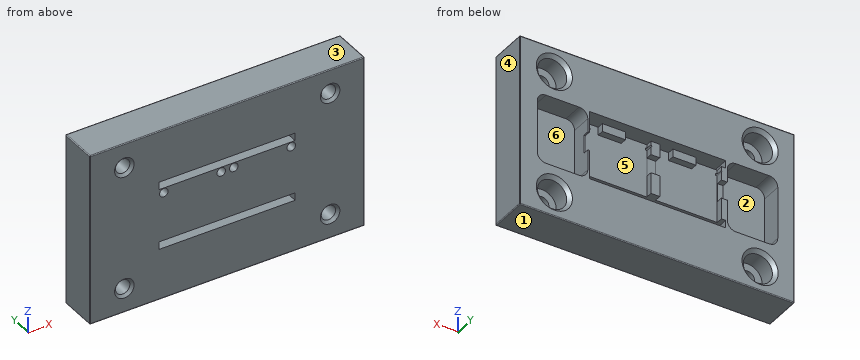
from build123d import *

# Parameters (mm, degrees)
SKETCH1_W             = 80.1116
SKETCH1_H             = 50.2158
BOSS_EXTRUDE1_DEPTH   = 11.176
HOLE1_D               = 4.191
HOLE1_CBORE_D         = 8.509
HOLE1_CBORE_DEPTH     = 5.7912
CHAMFER1_SIZE         = 1.016
FILLET1_R             = 0.254
CHAMFER2_SIZE         = 0.762
SKETCH4_W             = 39.751
SKETCH4_H             = 2.2352
CUT_EXTRUDE1_DEPTH    = 96.207132087
SKETCH5_R             = 1.2446
CUT_EXTRUDE2_DEPTH    = 4.2164
LPATTERN1_COUNT       = 2
LPATTERN1_PITCH       = 20.4216
F_1_0MM_DOWEL_HOLE1_D = 0.6858
SKETCH12_W            = 14.732
SKETCH12_H            = 20.32
CUT_EXTRUDE3_DEPTH    = 6.0198
FILLET2_R             = 2.54
CUT_EXTRUDE4_DEPTH    = 1.905
CUT_EXTRUDE5_REACH    = 81.263
SKETCH14_W            = 5.3848
SKETCH14_H            = 1.838231329


with BuildPart() as part:
    # Sketch1 → Boss-Extrude1 (new body)
    with BuildSketch(Plane(origin=(0, 0, 0), x_dir=(1, 0, 0), z_dir=(0, 1, 0))):
        with Locations((40.0558, 25.1079)):
            Rectangle(SKETCH1_W, SKETCH1_H)
    extrude(amount=BOSS_EXTRUDE1_DEPTH)

    # Hole1 (through all)
    with Locations(Plane(origin=(0, 11.176, 0), x_dir=(1, 0, 0), z_dir=(0, 1, 0))):
        with Locations((10.0457, 7.0993), (10.0584, 43.1419), (70.0532, 43.1292), (70.0532, 7.112)):
            CounterBoreHole(HOLE1_D / 2, HOLE1_CBORE_D / 2, HOLE1_CBORE_DEPTH)

    # Chamfer1
    chamfer1_edges = [part.edges().sort_by_distance(p)[0] for p in [
        (65.7987, 11.176, -7.112),
        (65.7987, 11.176, -43.1292),
        (5.8039, 11.176, -43.1419),
        (5.7912, 11.176, -7.0993),
    ]]
    chamfer(chamfer1_edges, length=CHAMFER1_SIZE)

    # Fillet1
    fillet1_edges = [part.edges().sort_by_distance(p)[0] for p in [
        (80.1116, 11.176, -25.1079),
        (40.0558, 11.176, -50.2158),
        (0, 11.176, -25.1079),
        (40.0558, 0, -50.2158),
        (80.1116, 0, -25.1079),
        (40.0558, 0, 0),
        (0, 0, -25.1079),
        (40.0558, 11.176, 0),
        (0, 5.588, -50.2158),
        (80.1116, 5.588, -50.2158),
        (80.1116, 5.588, 0),
        (0, 5.588, 0),
    ]]
    fillet(fillet1_edges, radius=FILLET1_R)

    # Chamfer2
    chamfer2_edges = [part.edges().sort_by_distance(p)[0] for p in [
        (72.1487, 0, -7.112),
        (72.1487, 0, -43.1292),
        (12.1539, 0, -43.1419),
        (12.1412, 0, -7.0993),
    ]]
    chamfer(chamfer2_edges, length=CHAMFER2_SIZE)

    # Sketch4 → Cut-Extrude1 (cut, through all)
    with BuildSketch(Plane.XZ):
        with Locations((39.9669, -16.3068)):
            Rectangle(SKETCH4_W, SKETCH4_H)
        with Locations((39.9669, -34.1122)):
            Rectangle(SKETCH4_W, SKETCH4_H)
    extrude(amount=-CUT_EXTRUDE1_DEPTH, mode=Mode.SUBTRACT)

    # Sketch5 → Cut-Extrude2 (cut)
    with BuildSketch(Plane.XZ):
        with Locations(Location((21.5646, -18.8214, 0), (0, 0, 270))):
            Circle(SKETCH5_R)
        with Locations(Location((38.3146, -18.8214, 0), (0, 0, 270))):
            Circle(SKETCH5_R)
    cut_extrude2 = extrude(amount=-CUT_EXTRUDE2_DEPTH, mode=Mode.SUBTRACT)

    # LPattern1: Cut-Extrude2 ×2
    with Locations(*[(i * LPATTERN1_PITCH, 0, 0) for i in range(1, LPATTERN1_COUNT)]):
        add(cut_extrude2, mode=Mode.SUBTRACT)

    # Ø1.0mm Dowel Hole1 (through all)
    with Locations(Plane(origin=(0, 4.2164, 0), x_dir=(-1, 0, 0), z_dir=(0, -1, 0))):
        with Locations((-21.5646, 18.8214), (-38.3146, 18.8214), (-41.9862, 18.8214), (-58.7362, 18.8214)):
            Hole(F_1_0MM_DOWEL_HOLE1_D / 2)

    # Sketch12 → Cut-Extrude3 (cut)
    with BuildSketch(Plane(origin=(0, 11.176, 0), x_dir=(1, 0, 0), z_dir=(0, 1, 0))):
        with Locations((12.2682, 25.1714)):
            Rectangle(SKETCH12_W, SKETCH12_H)
        with Locations((67.6656, 25.1714)):
            Rectangle(SKETCH12_W, SKETCH12_H)
    extrude(amount=-CUT_EXTRUDE3_DEPTH, mode=Mode.SUBTRACT)

    # Fillet2
    fillet2_edges = [part.edges().sort_by_distance(p)[0] for p in [
        (4.9022, 8.1661, -15.0114),
        (4.9022, 8.1661, -35.3314),
        (19.6342, 8.1661, -35.3314),
        (19.6342, 8.1661, -15.0114),
        (60.2996, 8.1661, -15.0114),
        (60.2996, 8.1661, -35.3314),
        (75.0316, 8.1661, -35.3314),
        (75.0316, 8.1661, -15.0114),
    ]]
    fillet(fillet2_edges, radius=FILLET2_R)

    # Sketch13 → Cut-Extrude4 (cut)
    with BuildSketch(Plane(origin=(0, 11.176, 0), x_dir=(1, 0, 0), z_dir=(0, 1, 0))):
        Polygon((28.7782, 19.7612), (35.5092, 19.7612), (35.5092, 17.4244), (39.3192, 17.4244), (39.3192, 19.7612), (39.3192, 32.9946), (21.336, 32.9946), (21.336, 19.7612), (21.336, 17.4244), (28.7782, 17.4244), align=None)
        Polygon((49.3268, 19.7612), (56.0578, 19.7612), (56.0578, 17.4244), (59.8678, 17.4244), (59.8678, 19.7612), (59.8678, 32.9946), (41.8846, 32.9946), (41.8846, 19.7612), (41.8846, 17.4244), (49.3268, 17.4244), align=None)
    extrude(amount=-CUT_EXTRUDE4_DEPTH, mode=Mode.SUBTRACT)

    # Cut-Extrude5: up to this face of the body (flat: up to its plane)
    cut_extrude5_end = Plane(part.part.faces().sort_by_distance((19.6342, 8.1661, -25.1714))[0])
    # Sketch14 → Cut-Extrude5 (cut, up to the picked face)
    with BuildSketch(Plane(origin=(60.2996, 0, 0), x_dir=(0, 0, -1), z_dir=(1, 0, 0)), mode=Mode.PRIVATE) as cut_extrude5_sk1:
        with Locations((24.13, 10.256884336)):
            Rectangle(SKETCH14_W, SKETCH14_H)
    cut_extrude5_tool1 = split(extrude(cut_extrude5_sk1.sketch, amount=-CUT_EXTRUDE5_REACH, mode=Mode.PRIVATE), bisect_by=cut_extrude5_end, keep=Keep.BOTH, mode=Mode.PRIVATE)
    add(cut_extrude5_tool1.solids().sort_by(Axis((60.2996, 10.256884, -24.13), (-1, 0, 0)))[0], mode=Mode.SUBTRACT)


solid = part.part
Could you check a few things on this model? Use its own coordinates, in mm. Face numbers are marked on the shaded views. A direction names the side the tool comes from. Give positions to 0.01 mm unless a question says otherwise; leave off trailing zeros. Write each loop counter-clockwise with the first axis right and the second up, starting at its lowest first coordinate (ties: lowest second). Pieces come first, ordered by that corner, then holes. Notation, with made-up numbers: (86, 50.25) -> (98, 50.25) arc R25 cw to (98, 80.25) -> close; hole circle Ø5 at (82.5, 11.5). An arc over 180 degrees is marked (long way). Write each question's results on one line, items separated by ' | '. Start each with the question number.
Q1. Suppose I cut it at A-A, the plane x = 44. List the corners of the cut face in (y, z) for me.
Q2. I need wall thicknesses on probe 1 along Z at (x, y) = (47.5, 8); probe 2 along Z at (x, y) = (10, 8.25); probe 3 along Z at (x, y) = (70, 6). Which ranges of each line are inside material? Lowest first, please.
Q3. Suppose I cut it at C-C, the plane x = 54.5. List the corners of the cut face in (y, z) for me.
Q4. I'm going to push flat-ended pins straight in: pin 1 Ø1.4 at (x, z) = (20.5, -25) entering from +Y; pin 2 Ø2.5 at (x, z) = (12, -7) entering from +Y. Where does each tip first touch, or does it pass through?
Q5. We'd pull the mould along Z, two halves only. Please class the marked faces 3, 4, 5 and 6: +Z half, -Z half, draft (parallel to the pull), parting line (faces both ways), or undercut.
Q6. Which directions (+Z, -Z, +X, -X, +Y, -Y) give clear straight access to the entire face, cutting with the end or side of a thin tool? Please do the marked faces 1 and 2.
Q7. Suppose I cut it at B-B, the plane y = 2.5. State how many separate pieces and enclosed holes the cut face has, and give its area (3 significant figures).
Outcome:
1) outline: (0, -49.96) arc R0.25 ccw to (0.25, -50.22) -> (10.92, -50.22) arc R0.25 ccw to (11.18, -49.96) -> (11.18, -35.23) -> (0, -35.23) -> close; (0, -32.99) -> (9.27, -32.99) -> (9.27, -17.42) -> (0, -17.42) -> close; (0, -15.19) -> (11.18, -15.19) -> (11.18, -0.25) arc R0.25 ccw to (10.92, 0) -> (0.25, 0) arc R0.25 ccw to (0, -0.25) -> close
2) probe 1: -50.22 to -35.23, -32.99 to -17.42, -15.19 to 0 | probe 2: -50.22 to -47.4, -38.89 to -35.33, -15.01 to -11.35, -2.85 to 0 | probe 3: -50.22 to -47.38, -38.88 to -35.33, -15.01 to -11.37, -2.86 to 0
3) outline: (0, -49.96) arc R0.25 ccw to (0.25, -50.22) -> (10.92, -50.22) arc R0.25 ccw to (11.18, -49.96) -> (11.18, -35.23) -> (0, -35.23) -> close; (0, -32.99) -> (9.27, -32.99) -> (9.27, -19.76) -> (11.18, -19.76) -> (11.18, -17.42) -> (0, -17.42) -> close; (0, -15.19) -> (11.18, -15.19) -> (11.18, -0.25) arc R0.25 ccw to (10.92, 0) -> (0.25, 0) arc R0.25 ccw to (0, -0.25) -> close
4) pin 1: y = 9.34 | pin 2: y = 5.38
5) face 3: +Z half | face 4: draft | face 5: undercut | face 6: undercut
6) face 1: -Z, +X, -X, +Y, -Y | face 2: +Y
7) separate pieces: 1 | enclosed holes: 10 | area: 3,770 mm2
